Autodesk Inventor part; units mm, degrees
ref_plane "YZ Plane" through (0, 0, 0) normal (1, 0, 0) x (0, 1, 0)
ref_plane "XZ Plane" through (0, 0, 0) normal (0, 1, 0) x (-1, 0, 0)
ref_plane "XY Plane" through (0, 0, 0) normal (0, 0, 1) x (1, 0, 0)
sketch "Skizze1" plane through (0, 0, 0) normal (0, 0, 1) x (1, 0, 0)
  circle A0 centre (0, 0) radius 6.3
  dimension "d0" = 12.6
extrude "Extrusion1" add sketch "Skizze1" along normal mid plane 22
sketch "Skizze2" plane through (0, 0, 11) normal (0, 0, 1) x (1, 0, 0)
  circle A0 centre (0, 0) radius 6.3
  circle A1 centre (0, 0) radius 4
  dimension "d3" = 8
extrude "Extrusion2" add sketch "Skizze2" along normal blind 24 contours A1
sketch "Skizze3" plane through (0, 0, 0) normal (1, 0, 0) x (0, 1, 0)
  circle A0 centre (0, 0) radius 1.1
  dimension "d6" = 2.2
extrude "Extrusion3" add sketch "Skizze3" along normal blind 26 and the other way blind 20
sketch "Skizze4" plane through (26, 0, 0) normal (1, 0, 0) x (0, 0, -1)
  circle A0 centre (0, 0) radius 0.3951
extrude "Extrusion4" add sketch "Skizze4" along normal blind 18
sketch "Skizze5" plane through (-20, 0, 0) normal (-1, 0, 0) x (0, 0, 1)
  circle A0 centre (0, 0) radius 0.6
  dimension "d13" = 1.2
extrude "Extrusion5" add sketch "Skizze5" along normal blind 22
properties part number "Probenkammer-Dummy" material "Glas"
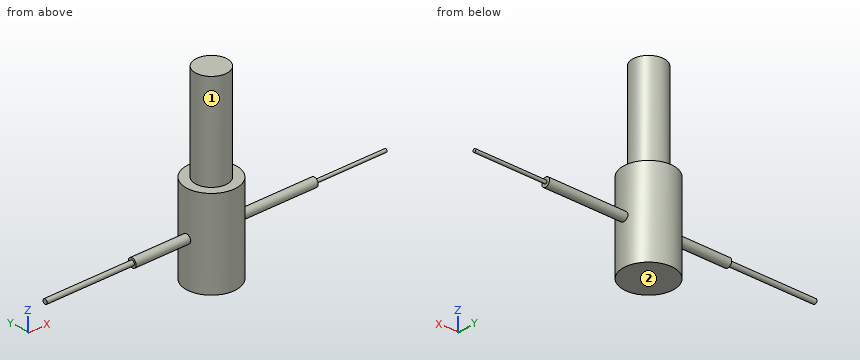
CAD build for the part. Positions are in the model's coordinates, mm. Face numbers are marked on the shaded views. A direction names the side the tool comes from. Give positions to 0.01 mm unless a question says otherwise; leave off trailing zeros. Order: outer loops, then holes, each group sorted by start corner. A loop starts at its lowest first (then second) coordinate and runs counter-clockwise, first axis right, second up. Notation, with made-up numbers: M 45,30.5 L 88,30.5 A6 ccw 88,41.5 Z; hole C 41,73.5 d7. An arc over 180 degrees is marked long. Put each result on its own line as item: value. Start each with the question number.
(1) Saw through at A-A, the plane x = 0. Write the cut outline in (y, z).
(2) Saw through at C-C, the plane z = 7.5. Write the cut outline in (x, y), then the cut area to 3 significant figures.
(3) Flat gauge pins, fed straight in: pin 1 Ø1 at (y, z) = (-2.5, 14.5) entering from +X; pin 2 Ø1.5 at (y, z) = (2.5, -1.5) entering from +X; pin 3 Ø4 at (x, z) = (-19.5, -1.5) entering from +Y. Where does each tip first touch, or does it go through?
(4) Which spindle directions (+Z, -Z, +X, -X, +Y, -Y) get a long thin tool onto all of the face, cutting with end or side? Do the marked faces 1 and 2. Say none if no direction does.
(5) Saw through at B-B, the plane z = 24.5. Write the cut outline in (x, y).
(6) Drill centre lines: line 1 along X through (y, z) = (0.5, -7); line 2 along Y through (x, z) = (-24, 0); line 3 along X through (y, z) = (0.25, 19.5). Where is each one in solid material? Low to high.
Check result:
1. outline: M -6.3,-11 L 6.3,-11 L 6.3,11 L 4,11 L 4,35 L -4,35 L -4,11 L -6.3,11 Z
2. outline: C 0,0 d12.6
2. area: 125 mm2
3. pin 1: stops at x = 3.46
3. pin 2: stops at x = 6.05
3. pin 3: stops at y = 1.1
4. face 1: +Z
4. face 2: -Z, +X, -X, +Y, -Y
5. outline: C 0,0 d8
6. line 1: x = -6.28 to 6.28
6. line 2: y = -0.6 to 0.6
6. line 3: x = -3.99 to 3.99
